```python
from build123d import *

# Parameters (mm, degrees)
F0_R          = 2.1666665
F1_DEPTH      = 5.5
F2_SIZE       = 0.75
F3_W          = 51
F3_H          = 8
F4_DEPTH      = 5.5
F5_SIZE       = 0.5
F6_W          = 2.5
F6_H          = 17
F7_DEPTH      = 12
F8_R          = 1.625
F9_DEPTH      = 25.301
F10_T1_DEPTH  = 2.5
F10_T3_DEPTH  = 2.5
F10_T8_DEPTH  = 17.5
F10_T14_DEPTH = 17.5
F10_T17_DEPTH = 17.5
F10_T19_DEPTH = 17.5
F11_R         = 5
F12_SIZE2     = 3
F12_SIZE      = 5
F12_2_SIZE2   = 3
F12_2_SIZE    = 5
F13_SIZE      = 1
F14_R         = 5
F15_SIZE2     = 2
F15_SIZE      = 3
F15_2_SIZE2   = 2
F15_2_SIZE    = 3
F16_T1_DEPTH  = 15.285841494
F16_T3_DEPTH  = 4.0033035506
F16_T5_DEPTH  = 4.0033035506
F17_R         = 1.7


# Not quite as in the source:
# - a fillet or chamfer that OpenCascade refuses, or shapes differently, is made with other operations: its cross-section is extruded or revolved along the edge and cut away or added


with BuildPart() as f1:
    # F0 (on Top) → F1 (new body)
    with BuildSketch(Plane.XY):
        with BuildLine():
            Line((25.5, 11), (-25.5, 11))
            Line((-25.5, 11), (-25.5, -11))
            Line((-25.5, -11), (-10.625, -11))
            Line((-10.625, -11), (-10.625, -0.125))
            ThreePointArc((-10.625, -0.125), (-4.5, 6), (1.625, -0.125))
            Line((1.625, -0.125), (1.625, -11))
            Line((1.625, -11), (25.5, -11))
            Line((25.5, -11), (25.5, 11))
        make_face()
        with Locations((-20.75, 0)):
            Circle(F0_R, mode=Mode.SUBTRACT)
        with Locations((21, 0)):
            Circle(F0_R, mode=Mode.SUBTRACT)
    extrude(amount=F1_DEPTH)

    # F2
    f2_edges = [f1.edges().sort_by_distance(p)[0] for p in [
        (-22.916666, 0, 0),
        (18.833334, 0, 0),
        (18.833334, 0, 5.5),
        (-22.916666, 0, 5.5),
    ]]
    chamfer(f2_edges, length=F2_SIZE)

    # F3 (on Top) → F4 (join, through all)
    with BuildSketch(Plane.XY):
        with Locations((0, 15)):
            Rectangle(F3_W, F3_H)
    extrude(amount=F4_DEPTH)

    # F5
    f5_edges = [f1.edges().sort_by_distance(p)[0] for p in [
        (-4.5, 6, 5.5),
        (-4.5, 6, 0),
        (-10.625, -5.5625, 5.5),
        (-10.625, -5.5625, 0),
        (1.625, -5.5625, 0),
        (1.625, -5.5625, 5.5),
    ]]
    chamfer(f5_edges, length=F5_SIZE)

    # F6 (on Top) → F7 (join)
    with BuildSketch(Plane.XY):
        with Locations((-7.55, 27.5)):
            Rectangle(F6_W, F6_H)
        with Locations((-1.45, 27.5)):
            Rectangle(F6_W, F6_H)
    extrude(amount=F7_DEPTH)

    # F8 (on face) → F9 (cut, through all)
    with BuildSketch(Plane.YZ.offset(-0.2)):
        with Locations((31, 7)):
            Circle(F8_R)
    extrude(amount=-F9_DEPTH, mode=Mode.SUBTRACT)

    # F10: fillet of radius 3 on 5 edges, made by hand

    # F10_s2 → F10_t1 (join)
    with BuildSketch(Plane.YZ.offset(-2.7)):
        with BuildLine():
            ThreePointArc((16, 5.5), (18.1213203436, 6.3786796564), (19, 8.5))
            Line((19, 8.5), (19, 5.5))
            Line((19, 5.5), (16, 5.5))
        make_face()
    extrude(amount=F10_T1_DEPTH)

    # F10_s4 → F10_t3 (join)
    with BuildSketch(Plane.YZ.offset(-8.8)):
        with BuildLine():
            ThreePointArc((16, 5.5), (18.1213203436, 6.3786796564), (19, 8.5))
            Line((19, 8.5), (19, 5.5))
            Line((19, 5.5), (16, 5.5))
        make_face()
    extrude(amount=F10_T3_DEPTH)


with BuildPart() as f10_tool6:
    # F10_s7 → F10_t8 (new body)
    with BuildSketch(Plane.YZ.offset(7.3)):
        with BuildLine():
            ThreePointArc((16, 5.5), (18.1213203436, 6.3786796564), (19, 8.5))
            Line((19, 8.5), (19, 5.5))
            Line((19, 5.5), (16, 5.5))
        make_face()
    extrude(amount=-F10_T8_DEPTH)

    split(bisect_by=Plane.YZ.offset(-6.3), keep=Keep.BOTTOM)

    split(bisect_by=Plane.YZ.offset(-8.8), keep=Keep.TOP)


with BuildPart() as f1_1:
    add(f1.part)

    # F10_t5: union F10_tool6
    add(f10_tool6.part)


with BuildPart() as f10_tool12:
    # F10_s13 → F10_t14 (new body)
    with BuildSketch(Plane.YZ.offset(1.2)):
        with BuildLine():
            ThreePointArc((16, 5.5), (18.1213203436, 6.3786796564), (19, 8.5))
            Line((19, 8.5), (19, 5.5))
            Line((19, 5.5), (16, 5.5))
        make_face()
    extrude(amount=-F10_T14_DEPTH)

    split(bisect_by=Plane.YZ.offset(-0.2), keep=Keep.BOTTOM)

    split(bisect_by=Plane.YZ.offset(-2.7), keep=Keep.TOP)


with BuildPart() as f1_2:
    add(f1_1.part)

    # F10_t11: union F10_tool12
    add(f10_tool12.part)

    # F10_s18 → F10_t17 (cut)
    with BuildSketch(Plane.YZ.offset(-10.2)):
        with BuildLine():
            ThreePointArc((19, 9), (19.8786796564, 11.1213203436), (22, 12))
            Line((22, 12), (19, 12))
            Line((19, 12), (19, 9))
        make_face()
    extrude(amount=F10_T17_DEPTH, mode=Mode.SUBTRACT)

    # F10_s20 → F10_t19 (cut)
    with BuildSketch(Plane.YZ.offset(-16.3)):
        with BuildLine():
            ThreePointArc((19, 9), (19.8786796564, 11.1213203436), (22, 12))
            Line((22, 12), (19, 12))
            Line((19, 12), (19, 9))
        make_face()
    extrude(amount=F10_T19_DEPTH, mode=Mode.SUBTRACT)

    # F11
    f11_edges = [f1_2.edges().sort_by_distance(p)[0] for p in [
        (-1.45, 36, 12),
        (-7.55, 36, 12),
    ]]
    fillet(f11_edges, radius=F11_R)

    # F12
    f12_edges = [f1_2.edges().sort_by_distance(p)[0] for p in [
        (-1.45, 36, 0),
    ]]
    f12_side = f1_2.faces().sort_by_distance((-1.45, 36, 3.5))[0]
    chamfer(f12_edges, length=F12_SIZE, length2=F12_SIZE2, reference=f12_side)

    # F12#2
    f12_2_edges = [f1_2.edges().sort_by_distance(p)[0] for p in [
        (-7.55, 36, 0),
    ]]
    f12_2_side = f1_2.faces().sort_by_distance((-7.55, 36, 3.5))[0]
    chamfer(f12_2_edges, length=F12_2_SIZE, length2=F12_2_SIZE2, reference=f12_2_side)

    # F13
    f13_edges = [f1_2.edges().sort_by_distance(p)[0] for p in [
        (-1.45, 36, 5),
        (-7.55, 36, 5),
    ]]
    chamfer(f13_edges, length=F13_SIZE)

    # F14
    f14_edges = [f1_2.edges().sort_by_distance(p)[0] for p in [
        (25.5, -11, 2.75),
        (-25.5, -11, 2.75),
        (25.5, 19, 2.75),
        (-25.5, 19, 2.75),
    ]]
    fillet(f14_edges, radius=F14_R)

    # F15
    f15_edges = [f1_2.edges().sort_by_distance(p)[0] for p in [
        (-10.625, -11, 2.75),
    ]]
    f15_side = f1_2.faces().sort_by_distance((-10.625, -5.5625, 2.75))[0]
    chamfer(f15_edges, length=F15_SIZE, length2=F15_SIZE2, reference=f15_side)

    # F15#2
    f15_2_edges = [f1_2.edges().sort_by_distance(p)[0] for p in [
        (1.625, -11, 2.75),
    ]]
    f15_2_side = f1_2.faces().sort_by_distance((11.08488, -11, 2.75))[0]
    chamfer(f15_2_edges, length=F15_2_SIZE, length2=F15_2_SIZE2, reference=f15_2_side)

    # F16: chamfer of 0.5 on 6 edges, made by hand

    # F16_s2 → F16_t1 (cut)
    with BuildSketch(Plane.XZ.offset(-34.285841494)):
        Polygon((-0.7, 0), (-0.2, 0.5), (-0.2, 0), align=None)
        Polygon((-2.2, 0), (-2.7, 0.5), (-2.7, 0), align=None)
        Polygon((-6.8, 0), (-6.3, 0.5), (-6.3, 0), align=None)
        Polygon((-8.3, 0), (-8.8, 0.5), (-8.8, 0), align=None)
    extrude(amount=F16_T1_DEPTH, mode=Mode.SUBTRACT)

    # F16_s4 → F16_t3 (cut)
    with BuildSketch(Plane.YZ.offset(-3.4516517753)):
        Polygon((32.7169048105, 0), (33.1456512734, 0.2427521223), (33, 0), align=None)
    extrude(amount=F16_T3_DEPTH, mode=Mode.SUBTRACT)

    # F16_s6 → F16_t5 (cut)
    with BuildSketch(Plane.YZ.offset(-9.5516517753)):
        Polygon((32.7169048105, 0), (33.1456512734, 0.2427521223), (33, 0), align=None)
    extrude(amount=F16_T5_DEPTH, mode=Mode.SUBTRACT)

    # F17
    f17_edges = [f1_2.edges().sort_by_distance(p)[0] for p in [
        (-8.8, 19, 3),
        (-6.3, 19, 3),
        (-2.7, 19, 3),
        (-0.2, 19, 3),
    ]]
    fillet(f17_edges, radius=F17_R)


solid = f1_2.part
```
Can you work these out from the model? Positions are in its coordinate system, mm. A direction names the side the tool comes from. Give positions to 0.01 mm unless a question says otherwise; leave off trailing zeros. Order: outer loops, then holes, each group sorted by start corner. A loop starts at its lowest first (then second) coordinate and runs counter-clockwise, first axis right, second up. Notation, with made-up numbers: M 51,54 L 83,54 A28 cw 83,86 Z; hole C 37.5,75.25 d7. An arc over 180 degrees is marked long. Write item = value, one per line. Start each with the question number.
Q1. Will these pins go through, and if not, where does the flat tip stop? pin 1 Ø3.5 at (x, y) = (21, 0) entering from +Z; pin 2 Ø6 at (x, z) = (15, 3) entering from +Y; pin 3 Ø6 at (y, z) = (23, 4) entering from +X; pin 4 Ø5 at (x, z) = (-5.5, 3) entering from +Y.
Q2. Suppose I cut it at A-A (y = 30). Write out the boundary of the cut face in (x, z), plus the area to 3 significant figures.
Q3. We'd pull the mould along Y, two halves only. Please class faces 6 (the flat face through (10, 19, 3)), 7 (the cylindrical face through (-1.432, 29.377, 7.071)), 8 (the flat face through (-8, 27, 12)), 9 (the cylindrical face through (-7.533, 29.377, 7.071)): pulls with the +Y half, pulls with the -Y half, needs draft (parallel to the pull), parting line crosses it, or undercut.
Q4. For faces 1 (the conical face through (-4.638, 6.134, 5.135)), 2 (the flat face through (-0.4, 25.7, 0.3)), 3 (the flat face through (-1.47, 34.3, 2.17)), 4 (the flat face through (-11.64, -9.52, 2.71)), 5 (the cylindrical face through (-3.211, 19.485, 3.035)), which set-ups out of +Z, -Z, +X, -X, +Y, -Y let a thin tool reach every point of the face, with its end or its side?
Q5. I need wall thicknesses on probe 1 along Z at (x, y) = (-1, 31) (3 decimals); probe 2 along X at (y, z) = (22.5, 5.75); probe 3 along Y at (x, z) = (-20.75, 3.8). Which ranges of each line are inside material? Lowest first, please. Write a range as [from, to].
Q6. Suppose I cut it at B-B (z = 10.25). Write out the boundary of the cut face in (x, y).
Q7. Suppose I cut it at D-D (y = 10). Write out the boundary of the cut face in (x, z), plus the area to 4 significant figures.
Q8. Suppose I cut it at C-C (x = 10.5). Write out the boundary of the cut face in (y, z).
Check result:
q1.pin_1 = through
q1.pin_2 = 19
q1.pin_3 = -0.05
q1.pin_4 = 35.83
q2.outline = M -8.8,0.5 L -8.3,0 L -6.8,0 L -6.3,0.5 L -6.3,5.72 L -8.8,5.72 Z; M -8.8,8.28 L -6.3,8.28 L -6.3,12 L -8.8,12 Z; M -2.7,0.5 L -2.2,0 L -0.7,0 L -0.2,0.5 L -0.2,5.72 L -2.7,5.72 Z; M -2.7,8.28 L -0.2,8.28 L -0.2,12 L -2.7,12 Z
q2.area = 46.7 mm2
q3.face_6 = pulls with the +Y half
q3.face_7 = undercut
q3.face_8 = needs draft
q3.face_9 = undercut
q4.face_1 = +Z, -Y
q4.face_2 = -Z, +X, +Y
q4.face_3 = -Z, +X, -X, +Y
q4.face_4 = +Z, -Z, -Y
q4.face_5 = +Z, -Z, +Y
q5.probe_1 = [0, 5.375], [8.625, 12]
q5.probe_2 = [-8.8, -6.3], [-2.7, -0.2]
q5.probe_3 = [-10.99, -2.17], [2.17, 18.99]
q6.outline = M -8.8,19.27 L -6.3,19.27 L -6.3,34.8 L -8.8,34.8 Z; M -2.7,19.27 L -0.2,19.27 L -0.2,34.8 L -2.7,34.8 Z
q7.outline = M -25.5,0 L 25.5,0 L 25.5,5.5 L -25.5,5.5 Z
q7.area = 280.5 mm2
q8.outline = M -11,0 L 19,0 L 19,5.5 L -11,5.5 Z
